Design review of the part built by this model. Coordinates are the model's own, in mm. A direction names the side the tool comes from. Give positions to 0.01 mm unless a question says otherwise; leave off trailing zeros. Loops run counter-clockwise (first coordinate to the right, second up) from the corner with the lowest first, then second, coordinate; pieces in that order, holes last. Notation, with made-up numbers: (-1, 89) - (24, 89) arc R21 ccw to (24, 126) - close; hole circle Ø9 at (-29.5, 66). An arc over 180 degrees is marked (long way). Write each question's results on one line, items separated by ' | '.
```python
from build123d import *

# Parameters (mm, degrees)
SKETCH1_R           = 1.5
BOSS_EXTRUDE1_DEPTH = 12.25
SKETCH2_R           = 2.5
BOSS_EXTRUDE2_DEPTH = 3
FILLET1_R           = 1
CHAMFER1_SIZE       = 0.25
CUT_EXTRUDE1_DEPTH  = 2


with BuildPart() as part:
    # Sketch1 → Boss-Extrude1 (new body)
    with BuildSketch(Plane(origin=(0, 0, 0), x_dir=(1, 0, 0), z_dir=(0, 1, 0))):
        with Locations(Location((0, 0, 0), (0, 0, 270))):
            Circle(SKETCH1_R)
    extrude(amount=BOSS_EXTRUDE1_DEPTH)

    # Sketch2 → Boss-Extrude2 (add)
    with BuildSketch(Plane(origin=(0, 12.25, 0), x_dir=(1, 0, 0), z_dir=(0, 1, 0))):
        with Locations(Location((0, 0, 0), (0, 0, 270))):
            Circle(SKETCH2_R)
    extrude(amount=BOSS_EXTRUDE2_DEPTH)

    # Fillet1
    fillet1_edges = [part.edges().sort_by_distance(p)[0] for p in [
        (0, 15.25, -2.5),
    ]]
    fillet(fillet1_edges, radius=FILLET1_R)

    # Chamfer1
    chamfer1_edges = [part.edges().sort_by_distance(p)[0] for p in [
        (0, 0, -1.5),
    ]]
    chamfer(chamfer1_edges, length=CHAMFER1_SIZE)

    # Sketch3 → Cut-Extrude1 (cut)
    with BuildSketch(Plane(origin=(0, 15.25, 0), x_dir=(1, 0, 0), z_dir=(0, 1, 0))):
        Polygon((-1, 0), (-0.5, -0.866025404), (0.5, -0.866025404), (1, 0), (0.5, 0.866025404), (-0.5, 0.866025404), align=None)
    extrude(amount=-CUT_EXTRUDE1_DEPTH, mode=Mode.SUBTRACT)


solid = part.part
```
Item 1: Clearance check with flat-ended pins moving along their axes: P1, Ø3, axis at x = -1.5, y = 11, coming from the -Z side; P2, Ø2, axis at x = -1.5, y = 9, coming from the +Z side; P3, Ø1.5, axis at y = 2, z = 1.5, coming from the -X side. State where each tip first meets the part, or that it passes through.
Output values:
P1: stops at z = -2.41 | P2: stops at z = 1.41 | P3: stops at x = -1.3
Item 2: We need section A-A on x = 0. Give the boundary of the cut face in (y, z), then the cut area to 3 significant figures.
Output values:
outline: (0, -1.25) - (0.25, -1.5) - (12.25, -1.5) - (12.25, -2.5) - (14.25, -2.5) arc R1 ccw to (15.25, -1.5) - (15.25, -0.87) - (13.25, -0.87) - (13.25, 0.87) - (15.25, 0.87) - (15.25, 1.5) arc R1 ccw to (14.25, 2.5) - (12.25, 2.5) - (12.25, 1.5) - (0.25, 1.5) - (0, 1.25) - close | area: 47.8 mm²
Item 3: Draft analysis for pull direction Z (two halves, no side actions). For faces 4 (the face through (-2, 12.25, 0)), 5 (the face through (0.75, 14.26, -0.43)), 6 (the face through (0, 14, -0.866)), 7 (the face through (-2.44, 13.24, -0.54)), state which applies: +Z half, -Z half, draft (parallel to the pull), parting line (faces both ways), or undercut.
Output values:
face 4: draft | face 5: undercut | face 6: undercut | face 7: parting line
Item 4: Wall thickness on probe 1 along Y at (x, z) = (0.65, -0.05); probe 2 along Y at (x, z) = (-1.6, -1.75); probe 3 along X at (y, z) = (5, -0.4): over which ranges is each line inside the solid? List them lowest first.
Output values:
probe 1: y = 0 to 13.25 | probe 2: y = 12.25 to 14.74 | probe 3: x = -1.45 to 1.45
Item 5: Tool access review of faces 1 (the face through (0.45, 6.17, 1.43)), 2 (the face through (-0.75, 14.26, 0.43)), 3 (the face through (0, 0, 0)): name each direction out of +Z, -Z, +X, -X, +Y, -Y from which nothing blocks a thin tool from reaching the whole face with its end or side.
Output values:
face 1: -Y | face 2: +Y | face 3: +Z, -Z, +X, -X, -Y
Item 6: We need section B-B on y = 1. Give the boundary of the cut face in (x, z).
Output values:
outline: circle Ø3 at (0, 0)
